Read the model definition and answer for the solid it produces. Units are mm, in the model's axes. A direction names the side the tool comes from. Give positions to 0.01 mm unless a question says otherwise; leave off trailing zeros. Write each loop counter-clockwise with the first axis right and the second up, starting at its lowest first coordinate (ties: lowest second). Pieces come first, ordered by that corner, then holes. Notation, with made-up numbers: (11, -1.75) - (39, -1.75) arc R16 ccw to (39, 24.25) - close; hole circle Ø10 at (-4.5, 15.5). An arc over 180 degrees is marked (long way). Answer as CSV lines item,"result".
```python
from build123d import *

# Parameters (mm, degrees)
F0_W     = 20
F0_H     = 3.05
F0_W_2   = 3.05
F0_H_2   = 10
F1_DEPTH = 3


with BuildPart() as f1:
    # F0 (on Front) → F1 (new body)
    with BuildSketch(Plane.XZ):
        Polygon((10, -11), (26.5, -11), (26.5, -5), (26.5, 5), (26.5, 11), (10, 11), (-10, 11), (-26.5, 11), (-26.5, 5), (-26.5, -5), (-26.5, -11), (-10, -11), align=None)
        with Locations((0, -12.525)):
            Rectangle(F0_W, F0_H)
        with Locations((28.025, 0)):
            Rectangle(F0_W_2, F0_H_2)
        with Locations((-28.025, 0)):
            Rectangle(F0_W_2, F0_H_2)
        with Locations((0, 12.525)):
            Rectangle(F0_W, F0_H)
    extrude(amount=F1_DEPTH)


solid = f1.part
```
(1) Find the intervals of material crossed by L1, parallel to Z at x = -24, y = -2.25; L2, parallel to X at y = -1.4, z = 10.75; L3, parallel to X at y = -2.65, z = 12.5, in increasing order.
Worked out:
L1,"z = -11 to 11"
L2,"x = -26.5 to 26.5"
L3,"x = -10 to 10"
(2) Each of these flat-tipped pins is pushed along its axis until it touches: P1, Ø1.5, axis at x = -17, y = -2, coming from the +Z side; P2, Ø1.5, axis at x = -28, y = -1.5, coming from the +Z side; P3, Ø0.9, axis at x = -18, y = -1, coming from the -Z side. Where does it stop, or does it pass through?
Worked out:
P1,"stops at z = 11"
P2,"stops at z = 5"
P3,"stops at z = -11"
(3) A cutting plane is placed at B-B (z = 9.75). Write down the section's boundary in (x, y).
Worked out:
outline,"(-26.5, -3) - (26.5, -3) - (26.5, 0) - (-26.5, 0) - close"
(4) A cutting plane is placed at C-C (x = 22.5). Write down the section's boundary in (y, z), and give its area (3 significant figures).
Worked out:
outline,"(-3, -11) - (0, -11) - (0, 11) - (-3, 11) - close"
area,"66.0 mm^2"
(5) For faces 1 (the flat face through (28, -1, 5)), 2 (the flat face through (18, -1, -11)), 3 (the flat face through (0, -1, 14.05)), 4 (the flat face through (-28, -1, -5)), 5 (the flat face through (-10, -1, 13)), determine the directions among +Z, -Z, +X, -X, +Y, -Y from which every point of the face is accessible in a straight line to the end or side of a thin tool.
Worked out:
face 1,"+Z, +X, +Y, -Y"
face 2,"-Z, +X, +Y, -Y"
face 3,"+Z, +X, -X, +Y, -Y"
face 4,"-Z, -X, +Y, -Y"
face 5,"+Z, -X, +Y, -Y"
(6) A cutting plane is placed at A-A (y = -1.3). Write down the section's boundary in (x, z).
Worked out:
outline,"(-29.55, -5) - (-26.5, -5) - (-26.5, -11) - (-10, -11) - (-10, -14.05) - (10, -14.05) - (10, -11) - (26.5, -11) - (26.5, -5) - (29.55, -5) - (29.55, 5) - (26.5, 5) - (26.5, 11) - (10, 11) - (10, 14.05) - (-10, 14.05) - (-10, 11) - (-26.5, 11) - (-26.5, 5) - (-29.55, 5) - close"
